Could you check a few things on this model? Use its own coordinates, in mm. Face numbers are marked on the shaded views. A direction names the side the tool comes from. Coordinates: 2 decimals unless noted, no trailing zeros. Loops run counter-clockwise (first coordinate to the right, second up) from the corner with the lowest first, then second, coordinate; pieces in that order, holes last.
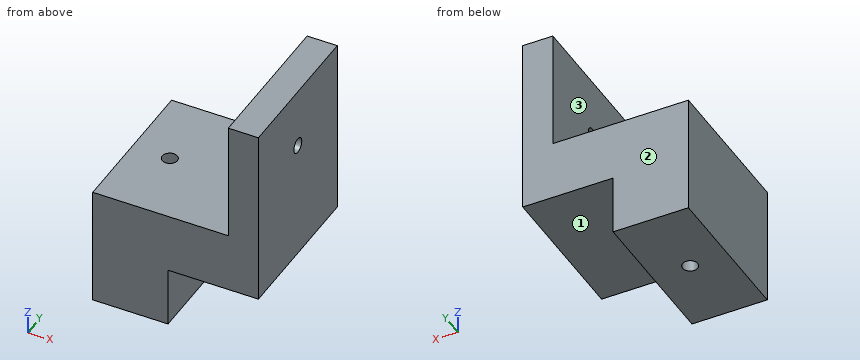
from build123d import *

# Parameters (mm, degrees)
CROQUIS1_W                                     = 25
CROQUIS1_H                                     = 50
SALIENTE_EXTRUIR1_DEPTH                        = 20
CROQUIS2_W                                     = 45
CROQUIS2_H                                     = 50
SALIENTE_EXTRUIR2_DEPTH                        = 20
CROQUIS5_W                                     = 20
CROQUIS5_H                                     = 50
CROQUIS5_W_2                                   = 40
SALIENTE_EXTRUIR3_DEPTH                        = 10
PERFORADOR_PARA_ROSCAR_PARA_MACHO_DE_ROS_D     = 5
PERFORADOR_PARA_ROSCAR_PARA_MACHO_DE_ROS_DEPTH = 11
PERFORADOR_PARA_ROSCAR_PARA_MACHO_DE_ROS_TIP   = 1.502151548
PERFORADOR_PARA_ROSCAR_PARA_MACHO_DE_2_D       = 5


with BuildPart() as part:
    # Croquis1 → Saliente-Extruir1 (new body)
    with BuildSketch(Plane.XY):
        with Locations((-28.587290739, 5.380089213)):
            Rectangle(CROQUIS1_W, CROQUIS1_H)
    extrude(amount=SALIENTE_EXTRUIR1_DEPTH)

    # Croquis2 → Saliente-Extruir2 (add)
    with BuildSketch(Plane.XY.offset(20)):
        with Locations((-18.587290739, 5.380089213)):
            Rectangle(CROQUIS2_W, CROQUIS2_H)
    extrude(amount=SALIENTE_EXTRUIR2_DEPTH)

    # Croquis5 → Saliente-Extruir3 (add)
    with BuildSketch(Plane(origin=(3.912709261, 0, 0), x_dir=(0, 0, -1), z_dir=(1, 0, 0))):
        with Locations((-30, 5.380089213)):
            Rectangle(CROQUIS5_W, CROQUIS5_H)
        with Locations((-60, 5.380089213)):
            Rectangle(CROQUIS5_W_2, CROQUIS5_H)
    extrude(amount=SALIENTE_EXTRUIR3_DEPTH)

    # Perforador para roscar para macho de ros
    with Locations(Plane(origin=(3.912709261, 5.380089213, 60), x_dir=(0, 0, -1), z_dir=(-1, 0, 0))):
        with Locations((0, 0)):
            Hole(PERFORADOR_PARA_ROSCAR_PARA_MACHO_DE_ROS_D / 2, depth=PERFORADOR_PARA_ROSCAR_PARA_MACHO_DE_ROS_DEPTH)
            with Locations((0, 0, -(PERFORADOR_PARA_ROSCAR_PARA_MACHO_DE_ROS_DEPTH + PERFORADOR_PARA_ROSCAR_PARA_MACHO_DE_ROS_TIP / 2))):  # 118° drill point
                Cone(0, PERFORADOR_PARA_ROSCAR_PARA_MACHO_DE_ROS_D / 2, PERFORADOR_PARA_ROSCAR_PARA_MACHO_DE_ROS_TIP, mode=Mode.SUBTRACT)

    # Perforador para roscar para macho de 2 (through all)
    with Locations(Plane(origin=(-28.587290739, 5.380089213, 0), x_dir=(-1, 0, 0), z_dir=(0, 0, -1))):
        with Locations((0, 0)):
            Hole(PERFORADOR_PARA_ROSCAR_PARA_MACHO_DE_2_D / 2)


solid = part.part
(1) Which directions (+Z, -Z, +X, -X, +Y, -Y) give clear straight access to the entire face, cutting with the end or side of a thin tool? Please do the marked faces 1, 2 and 3.
Answers:
face 1: -Z, +X, +Y, -Y
face 2: +Z, -Z, +X, -X, +Y
face 3: +Z, -X, +Y, -Y
(2) Imagine slicing it at A-A, the plane z = 60. Write out the boundary of the cut face in (x, y).
Answers:
outline: (3.91, -19.62) - (13.91, -19.62) - (13.91, 2.88) - (3.91, 2.88) - close; (3.91, 7.88) - (13.91, 7.88) - (13.91, 30.38) - (3.91, 30.38) - close
(3) Imagine slicing it at C-C, the plane z = 72. Write out the boundary of the cut face in (x, y), and give its area (3 significant figures).
Answers:
outline: (3.91, -19.62) - (13.91, -19.62) - (13.91, 30.38) - (3.91, 30.38) - close
area: 500 mm2
(4) For pin 1 (4 mm diameter, centred on x = -28.59, y = 5.38, fed in from -Z); pin 2 (12 mm diameter, centred on y = -6, z = 53.5, fed in from -X); pin 3 (5 mm diameter, centred on x = -8.5, y = -12, fed in from -Z); pin 4 (4 mm diameter, centred on x = -29.5, y = 18.5, fed in from +Z), each with a flat end and sliding along its axis, tell me the tip position at first contact or that it passes through.
Answers:
pin 1: passes through
pin 2: stops at x = 3.91
pin 3: stops at z = 20
pin 4: stops at z = 40
(5) Imagine slicing it at B-B, the plane y = -8. Write out the boundary of the cut face in (x, z).
Answers:
outline: (-41.09, 0) - (-16.09, 0) - (-16.09, 20) - (13.91, 20) - (13.91, 80) - (3.91, 80) - (3.91, 40) - (-41.09, 40) - close
(6) I need wall thicknesses on probe 1 along Y at (x, z) = (9.25, 60); probe 2 along Z at (x, y) = (-12, -8); probe 3 along Y at (x, z) = (-28, 39.5). Which ranges of each line are inside material? Lowest first, please.
Answers:
probe 1: y = -19.62 to 2.88, 7.88 to 30.38
probe 2: z = 20 to 40
probe 3: y = -19.62 to 2.95, 7.81 to 30.38
(7) Imagine slicing it at D-D, the plane x = -6. Write out the boundary of the cut face in (y, z), and give its area (3 significant figures).
Answers:
outline: (-19.62, 20) - (30.38, 20) - (30.38, 40) - (-19.62, 40) - close
area: 1,000 mm2
